```python
from build123d import *

# Parameters (mm, degrees)
SKETCH1_W               = 30.562599784
SKETCH1_H               = 30.562599784
BOSS_EXTRUDE1_DEPTH     = 139.7
CUT_EXTRUDE1_DEPTH      = 142.361685943
CUT_EXTRUDE1_DEPTH_BACK = 142.361685943
BOSS_EXTRUDE2_DEPTH     = 5.09983
SKETCH5_R               = 1.8
CUT_EXTRUDE2_DEPTH      = 146.354775845
SKETCH6_R               = 1.662500104
CUT_EXTRUDE3_DEPTH      = 145.138064655
BOSS_EXTRUDE3_REACH     = 212.94
BOSS_EXTRUDE3_START     = 66.802
SKETCH8_W               = 34.925
SKETCH8_H               = 34.925
SKETCH8_W_2             = 30.562599784
SKETCH8_H_2             = 30.562599784


with BuildPart() as part:
    # Sketch1 → Boss-Extrude1 (new body)
    with BuildSketch(Plane(origin=(0, 0, 0), x_dir=(1, 0, 0), z_dir=(0, 1, 0))):
        Rectangle(SKETCH1_W, SKETCH1_H)
    extrude(amount=BOSS_EXTRUDE1_DEPTH)

    # Sketch2 → Cut-Extrude1 (cut, two sides: drawn at the far end of the back side and taken through both)
    with BuildSketch(Plane(origin=(0, 0, 0), x_dir=(0, -1, 0), z_dir=(-0.7071067811865438, 0, -0.7071067811865512)).offset(-CUT_EXTRUDE1_DEPTH_BACK)):
        Polygon((-139.7, -5.11931044), (-81.186013921, 0), (-79.295294527, -21.611021558), (-139.7, -21.611021558), align=None)
    extrude(amount=CUT_EXTRUDE1_DEPTH + CUT_EXTRUDE1_DEPTH_BACK, mode=Mode.SUBTRACT)

    # Sketch4 → Boss-Extrude2 (add)
    with BuildSketch(Plane(origin=(-4.984326181, 0.616698988, 4.984326181), x_dir=(-0.6990962056889038, 0.08640854919208918, -0.7097873328102555), z_dir=(0.7044160264027624, -0.08715574274765817, -0.704416026402755))):
        Polygon((40.57727892, 136.609827857), (-16.357328672, 141.566939751), (-21.314440566, 84.632332159), (35.620167026, 79.675220265), align=None)
    extrude(amount=-BOSS_EXTRUDE2_DEPTH)

    # Sketch5 → Cut-Extrude2 (cut, through all)
    with BuildSketch(Plane(origin=(-4.984326181, 0.616698988, 4.984326181), x_dir=(-0.6990962056889037, 0.0864085491920891, -0.7097873328102555), z_dir=(0.7044160264027625, -0.08715574274765821, -0.7044160264027549))):
        with Locations(Location((33.998237872, 131.084660992, 0), (0, 0, 355.023990467))):
            Circle(SKETCH5_R)
        with Locations(Location((-10.832161807, 134.987898703, 0), (0, 0, 355.023990467))):
            Circle(SKETCH5_R)
        with Locations(Location((-14.735399518, 90.157499024, 0), (0, 0, 355.023990467))):
            Circle(SKETCH5_R)
        with Locations(Location((30.095000161, 86.254261313, 0), (0, 0, 355.023990467))):
            Circle(SKETCH5_R)
        Polygon((19.811839734, 123.787667921), (9.849528694, 124.65505408), (9.329097, 118.677667456), (19.291408039, 117.810281298), align=None)
    extrude(amount=-CUT_EXTRUDE2_DEPTH, mode=Mode.SUBTRACT)

    # Sketch6 → Cut-Extrude3 (cut, symmetric)
    with BuildSketch(Plane(origin=(0, 0, 0), x_dir=(0, 0, -1), z_dir=(1, 0, 0))):
        with Locations(Location((0, 25.4, 0), (0, 0, 180))):
            Circle(SKETCH6_R)
        with Locations(Location((-9.5, 15.9, 0), (0, 0, 180))):
            Circle(SKETCH6_R)
        with Locations(Location((9.5, 15.9, 0), (0, 0, 180))):
            Circle(SKETCH6_R)
        with Locations(Location((0, 6.4, 0), (0, 0, 180))):
            Circle(SKETCH6_R)
    cut_extrude3 = extrude(amount=CUT_EXTRUDE3_DEPTH, both=True, mode=Mode.SUBTRACT)

    # Mirror1: Cut-Extrude3 across plane
    add(cut_extrude3.mirror(Plane(origin=(0, 0, 0), x_dir=(-0.7071067811865512, 0, 0.7071067811865439), z_dir=(-0.7071067811865438, 0, -0.7071067811865512))), mode=Mode.SUBTRACT)

    # Boss-Extrude3: up to this plane
    boss_extrude3_end = Plane(origin=(15.281299892, 81.186013921, 15.281299892), z_dir=(-0.06162841671621989, -0.9961946980917455, 0.061628416716219235))
    # Sketch8 → Boss-Extrude3 (add, up to the surface)
    with BuildSketch(Plane(origin=(0, 0, 0), x_dir=(1, 0, 0), z_dir=(0, 1, 0)).offset(BOSS_EXTRUDE3_START), mode=Mode.PRIVATE) as boss_extrude3_sk1:
        Rectangle(SKETCH8_W, SKETCH8_H)
        Rectangle(SKETCH8_W_2, SKETCH8_H_2, mode=Mode.SUBTRACT)
    boss_extrude3_tool1 = split(extrude(boss_extrude3_sk1.sketch, amount=BOSS_EXTRUDE3_REACH, mode=Mode.PRIVATE), bisect_by=boss_extrude3_end, keep=Keep.BOTH, mode=Mode.PRIVATE)
    add(boss_extrude3_tool1.solids().sort_by_distance((0, 66.802, 16.968586))[0])


solid = part.part
```
Part model, mm, in its own coordinate system. A direction names the side the tool comes from. Coordinates: 2 decimals unless noted, no trailing zeros. Order: outer loops, then holes, each group sorted by start corner. A loop starts at its lowest first (then second) coordinate and runs counter-clockwise, first axis right, second up. Notation, with made-up numbers: (20.25, 37.5) - (73.25, 37.5) arc R11 ccw to (73.25, 47.5) - close; hole circle Ø8 at (-13.75, -34.5). An arc over 180 degrees is marked (long way). Return JSON: item names as keys, results as strings. Group by question number.
Item 1: Cut at A-A (y = 6.4). List the corners of the cut face in (x, z).
Item 2: Drill centre lines: probe 1 along Z at (x, y) = (-11.25, 15.9); probe 2 along Y at (x, z) = (0, -5); probe 3 along X at (y, z) = (15, 4). Where is each one in solid material? Low to high. Write a range as from..to.
Item 3: Cut at C-C (z = 5.5). List the corners of the cut face in (x, y) (1 decimal), plus the area to 3 significant figures.
Item 4: Pull direction Z, two halves, no side cores. Call faces 6 (the face through (-16, 66.802, 0)), 7 (the face through (0.133, 16.537, -7.964)), 8 (the face through (0, 74, -17.462)), 9 (the face through (14.887, 90.816, 17.264)): pulls with the +Z half, pulls with the -Z half, needs draft (parallel to the pull), parting line crosses it, or undercut.
Item 5: Cut at B-B (x = 5.5). List the corners of the cut face in (y, z) (1 decimal), plus the area to 3 significant figures.
Item 6: Which spindle directions (+Z, -Z, +X, -X, +Y, -Y) get a long thin tool onto all of the face, cutting with end or side? Do faces 1 (the face through (-7, 139.7, 7)), 2 (the face through (0, 33, -15.281)), 3 (the face through (0, 33, 15.281)), 4 (the face through (17.462, 74, 0)), 5 (the face through (-9.57, 122.86, -3.16)). Say none if no direction does.
Item 7: Cut at D-D (y = 51.5). List the corners of the cut face in (x, z), plus the area to 3 significant figures.
Item 8: Pin check, flat tips, straight feed: pin 1 (3 mm diameter, centred on x = -10, z = 13, fed in from +Y); pin 2 (4 mm diameter, centred on x = 9.5, y = 15.9, fed in from -Z); pin 3 (8 mm diameter, centred on y = 24, z = -16.5, fed in from +X). Stop position of each tip, or through.
Check values:
{
 "1": {"outline": "(-15.28, -15.28) - (-1.66, -15.28) - (-1.66, -1.66) - (-15.28, -1.66) - close; (-15.28, 1.66) - (-1.66, 1.66) - (-1.66, 15.28) - (-15.28, 15.28) - close; (1.66, -15.28) - (15.28, -15.28) - (15.28, -1.66) - (1.66, -1.66) - close; (1.66, 1.66) - (15.28, 1.66) - (15.28, 15.28) - (1.66, 15.28) - close"},
 "2": {"probe 1": "z = -15.28..-11.16, -7.84..7.84, 11.16..15.28", "probe 2": "y = 0..4.74, 8.06..23.74, 27.06..80.88, 125.21..139.84", "probe 3": "x = -15.28..-10.9, -8.1..8.1, 10.9..15.28"},
 "3": {"outline": "(-17.5, 66.8) - (-15.3, 66.8) - (-15.3, 0) - (15.3, 0) - (15.3, 66.8) - (17.5, 66.8) - (17.5, 80.4) - (5.5, 81.2) - (12.7, 139.7) - (5.6, 140.1) - (5.5, 139.7) - (-15.3, 139.7) - (-15.3, 126.8) - (-4.1, 126.1) - (-4.1, 120.1) - (-15.3, 120.8) - (-15.3, 82.5) - (-17.5, 82.6) - close; hole circle Ø3.3 at (-9.5, 15.9); hole circle Ø3.3 at (0, 6.4); hole circle Ø3.3 at (0, 25.4); hole circle Ø3.3 at (9.5, 15.9)", "area": "3,870 mm2"},
 "4": {"face 6": "needs draft", "face 7": "undercut", "face 8": "pulls with the -Z half", "face 9": "undercut"},
 "5": {"outline": "(0, -15.3) - (66.8, -15.3) - (66.8, -17.5) - (79.8, -17.5) - (81.2, 5.5) - (139.7, -1.7) - (140.1, 5.4) - (139.7, 5.5) - (139.7, 15.3) - (81.8, 15.3) - (81.9, 17.5) - (66.8, 17.5) - (66.8, 15.3) - (0, 15.3) - close; hole circle Ø3.3 at (6.4, 0); hole circle Ø3.3 at (15.9, -9.5); hole circle Ø3.3 at (15.9, 9.5); hole circle Ø3.3 at (25.4, 0)", "area": "3,280 mm2"},
 "6": {"face 1": "+Z, -X, +Y", "face 2": "-Z, +X, -X, -Y", "face 3": "+Z, +X, -X, -Y", "face 4": "+Z, -Z, +X, -Y", "face 5": "none"},
 "7": {"outline": "(-15.28, -15.28) - (15.28, -15.28) - (15.28, 15.28) - (-15.28, 15.28) - close", "area": "934 mm2"},
 "8": {"pin 1": "stops at y = 139.7", "pin 2": "stops at z = -15.28", "pin 3": "stops at x = 15.28"}
}
